from build123d import *

# Parameters (mm, degrees)
BOSS_EXTRUDE2_DEPTH = 8
SKETCH5_R           = 2.1
CUT_EXTRUDE1_DEPTH  = 130.846239099
FILLET1_R           = 8
SKETCH6_R           = 1
CUT_EXTRUDE2_DEPTH  = 7
BOSS_EXTRUDE3_DEPTH = 10
FILLET2_R           = 2
SKETCH9_W           = 4
SKETCH9_H           = 4
BOSS_EXTRUDE4_DEPTH = 21
SKETCH10_W          = 34
SKETCH10_H          = 4
BOSS_EXTRUDE5_DEPTH = 4
FILLET3_R           = 2
FILLET4_R           = 1
SKETCH11_R          = 1.95
CUT_EXTRUDE3_DEPTH  = 132.988809405


with BuildPart() as part:
    # Sketch3 → Boss-Extrude2 (new body)
    with BuildSketch(Plane(origin=(0, 0, 0), x_dir=(1, 0, 0), z_dir=(0, 1, 0))):
        Polygon((-66.423008775, -50), (-66.423008775, 50), (-15, 111.28355545), (15, 111.28355545), (66.423008775, 50), (66.423008775, -50), (15, -111.28355545), (-15, -111.28355545), align=None)
    extrude(amount=BOSS_EXTRUDE2_DEPTH)

    # Sketch5 → Cut-Extrude1 (cut, through all)
    with BuildSketch(Plane(origin=(0, 8, 0), x_dir=(1, 0, 0), z_dir=(0, 1, 0))):
        with Locations(Location((0, -106.28355545, 0), (0, 0, 270))):
            Circle(SKETCH5_R)
        with Locations(Location((-61.423008775, -48.180148829, 0), (0, 0, 270))):
            Circle(SKETCH5_R)
        with Locations(Location((0, 106.28355545, 0), (0, 0, 90))):
            Circle(SKETCH5_R)
        with Locations(Location((-61.423008775, 48.180148829, 0), (0, 0, 90))):
            Circle(SKETCH5_R)
        with Locations(Location((61.423008775, 48.180148829, 0), (0, 0, 270))):
            Circle(SKETCH5_R)
        with Locations(Location((61.423008775, -48.180148829, 0), (0, 0, 90))):
            Circle(SKETCH5_R)
    extrude(amount=-CUT_EXTRUDE1_DEPTH, mode=Mode.SUBTRACT)

    # Fillet1
    fillet1_edges = [part.edges().sort_by_distance(p)[0] for p in [
        (-66.423008775, 4, 50),
        (-66.423008775, 4, -50),
        (-15, 4, -111.28355545),
        (15, 4, -111.28355545),
        (66.423008775, 4, -50),
        (66.423008775, 4, 50),
        (15, 4, 111.28355545),
        (-15, 4, 111.28355545),
    ]]
    fillet(fillet1_edges, radius=FILLET1_R)

    # Sketch6 → Cut-Extrude2 (cut)
    with BuildSketch(Plane(origin=(0, 8, 0), x_dir=(1, 0, 0), z_dir=(0, 1, 0))):
        with Locations(Location((-44.948008775, -3.34355545, 0), (0, 0, 270))):
            Circle(SKETCH6_R)
        with Locations(Location((-44.948008775, -59.22355545, 0), (0, 0, 270))):
            Circle(SKETCH6_R)
        with Locations(Location((-25.898008775, -59.22355545, 0), (0, 0, 90))):
            Circle(SKETCH6_R)
        with Locations(Location((-25.898008775, -3.34355545, 0), (0, 0, 90))):
            Circle(SKETCH6_R)
        with Locations(Location((44.948008775, -59.22355545, 0), (0, 0, 90))):
            Circle(SKETCH6_R)
        with Locations(Location((25.898008775, -59.22355545, 0), (0, 0, 270))):
            Circle(SKETCH6_R)
        with Locations(Location((44.948008775, -3.34355545, 0), (0, 0, 90))):
            Circle(SKETCH6_R)
        with Locations(Location((25.898008775, -3.34355545, 0), (0, 0, 270))):
            Circle(SKETCH6_R)
    extrude(amount=-CUT_EXTRUDE2_DEPTH, mode=Mode.SUBTRACT)

    # Sketch8 → Boss-Extrude3 (add)
    with BuildSketch(Plane(origin=(0, 8, 0), x_dir=(1, 0, 0), z_dir=(0, 1, 0))):
        Polygon((8.295310149, 79.28355545), (11.295310149, 79.28355545), (11.295310149, 8.28355545), (29.895310149, 8.28355545), (29.895310149, 79.28355545), (32.895310149, 79.28355545), (32.895310149, 5.28355545), (8.295310149, 5.28355545), align=None)
    extrude(amount=BOSS_EXTRUDE3_DEPTH)

    # Fillet2
    fillet2_edges = [part.edges().sort_by_distance(p)[0] for p in [
        (8.295310149, 8, -42.28355545),
        (20.595310149, 8, -5.28355545),
        (32.895310149, 8, -42.28355545),
        (31.395310149, 8, -79.28355545),
        (9.795310149, 8, -79.28355545),
    ]]
    fillet(fillet2_edges, radius=FILLET2_R)

    # Sketch9 → Boss-Extrude4 (add)
    with BuildSketch(Plane(origin=(0, 8, 0), x_dir=(1, 0, 0), z_dir=(0, 1, 0))):
        with Locations((-44.423008775, 41.28355545)):
            Rectangle(SKETCH9_W, SKETCH9_H)
        with Locations((-14.423008775, 41.28355545)):
            Rectangle(SKETCH9_W, SKETCH9_H)
    extrude(amount=BOSS_EXTRUDE4_DEPTH)

    # Sketch10 → Boss-Extrude5 (add)
    with BuildSketch(Plane(origin=(0, 29, 0), x_dir=(1, 0, 0), z_dir=(0, 1, 0))):
        with Locations((-29.423008775, 41.28355545)):
            Rectangle(SKETCH10_W, SKETCH10_H)
    extrude(amount=BOSS_EXTRUDE5_DEPTH)

    # Fillet3
    fillet3_edges = [part.edges().sort_by_distance(p)[0] for p in [
        (-44.423008775, 8, -43.28355545),
        (-46.423008775, 8, -41.28355545),
        (-44.423008775, 8, -39.28355545),
        (-12.423008775, 8, -41.28355545),
        (-14.423008775, 8, -43.28355545),
        (-14.423008775, 8, -39.28355545),
        (-46.423008775, 33, -41.28355545),
        (-12.423008775, 33, -41.28355545),
    ]]
    fillet(fillet3_edges, radius=FILLET3_R)

    # Fillet4
    fillet4_edges = [part.edges().sort_by_distance(p)[0] for p in [
        (8.295310149, 18, -42.28355545),
        (20.595310149, 18, -5.28355545),
        (32.895310149, 18, -42.28355545),
    ]]
    fillet(fillet4_edges, radius=FILLET4_R)

    # Sketch11 → Cut-Extrude3 (cut, through all)
    with BuildSketch(Plane(origin=(0, 8, 0), x_dir=(1, 0, 0), z_dir=(0, 1, 0))):
        with Locations(Location((12.2, 0, 0), (0, 0, 270))):
            Circle(SKETCH11_R)
        with Locations(Location((-12.2, 0, 0), (0, 0, 270))):
            Circle(SKETCH11_R)
    extrude(amount=-CUT_EXTRUDE3_DEPTH, mode=Mode.SUBTRACT)


solid = part.part
Input: part model. Units: mm. Frame: model coordinates. A direction names the side the tool comes from. Coordinates: 2 decimals unless noted, no trailing zeros. Order: outer loops, then holes, each group sorted by start corner. A loop starts at its lowest first (then second) coordinate and runs counter-clockwise, first axis right, second up. Notation, with made-up numbers: M -11,80.25 L -4,80.25 A6 ccw -4,90.25 Z; hole C 17,-30.5 d2. An arc over 180 degrees is marked long. One line per question, with ' | ' between items.
Item 1: Section B-B (y = 13). Output: boundary loops of the cut face in (x, z), then the cut area to 3 significant figures.
Geometry results:
outline: M -46.42,-43.28 L -42.42,-43.28 L -42.42,-39.28 L -46.42,-39.28 Z; M -16.42,-43.28 L -12.42,-43.28 L -12.42,-39.28 L -16.42,-39.28 Z; M 8.3,-79.28 L 11.3,-79.28 L 11.3,-8.28 L 29.9,-8.28 L 29.9,-79.28 L 32.9,-79.28 L 32.9,-5.28 L 8.3,-5.28 Z | area: 532 mm^2
Item 2: Reachability of faces 1 (the flat face through (-42.423, 18, -41)), 2 (the cylindrical face through (-65.954, 4.056, -49.788)), 3 (the flat face through (-46.423, 20, -41)), 4 (the flat face through (20, 13, -8.284)), 5 (the flat face through (-30, 32, -39.284)) from +Z, -Z, +X, -X, +Y, -Y: full face, straight path, thin tool, end or side. Return the list, or none.
Geometry results:
face 1: +Z, -Z | face 2: -Z, -X, +Y, -Y | face 3: +Z, -Z, -X, +Y | face 4: -Z, +Y | face 5: +Z, -X, +Y
Item 3: Pin query (flat end, axial travel): pin 1 (10 mm diameter, centred on x = 2.5, y = 11, fed in from +Z); pin 2 (2.5 mm diameter, centred on y = 15, z = -40.5, fed in from -X); pin 3 (10 mm diameter, centred on x = 35.5, y = 20.5, fed in from +Z); pin 4 (6.5 mm diameter, centred on x = -61.42, z = -48.18, fed in from +Y). Return the tip coordinate at first contact, or that it passes through.
Geometry results:
pin 1: stops at z = 111.28 | pin 2: stops at x = -46.42 | pin 3: stops at z = -5.28 | pin 4: stops at y = 8
Item 4: Section D-D (z = -67). Output: boundary loops of the cut face in (x, y), then the cut area to 3 significant figures.
Geometry results:
outline: M -52.16,0 L 52.16,0 L 52.16,8 L 34.9,8 A2 cw 32.9,10 L 32.9,17 A1 ccw 31.9,18 L 29.9,18 L 29.9,8 L 11.3,8 L 11.3,18 L 9.3,18 A1 ccw 8.3,17 L 8.3,10 A2 cw 6.3,8 L -52.16,8 Z | area: 896 mm^2
Item 5: Draft query along Z for faces 6 (the flat face through (1, 0, -2)), 7 (the flat face through (21, 13, -5.284)), 8 (the cylindrical face through (63.47, 4.06, 48.64)), 9 (the cylindrical face through (-63.505, 4.056, -47.907)). Return one class per face: released by +Z, released by -Z, zero draft, split by the parting line, or undercut.
Geometry results:
face 6: zero draft | face 7: released by +Z | face 8: undercut | face 9: undercut
Item 6: Section C-C (y = 26.5). Output: boundary loops of the cut face in (x, z).
Geometry results:
outline: M -46.42,-43.28 L -42.42,-43.28 L -42.42,-39.28 L -46.42,-39.28 Z; M -16.42,-43.28 L -12.42,-43.28 L -12.42,-39.28 L -16.42,-39.28 Z
Item 7: Ray query, line 1 along X through (y, z) = (5, 4); line 2 along Y through (x, z) = (-60.5, 11.5); line 3 along Z through (x, y) = (19, 14.5). Return the intervals inside material, ascending.
Geometry results:
line 1: x = -66.42 to -45.7, -44.19 to -26.65, -25.14 to 25.14, 26.65 to 44.19, 45.7 to 66.42 | line 2: y = 0 to 8 | line 3: z = -8.28 to -5.28
Item 8: Section A-A (x = 0). Output: boundary loops of the cut face in (y, z).
Geometry results:
outline: M 0,-111.28 L 8,-111.28 L 8,-108.38 L 0,-108.38 Z; M 0,-104.18 L 8,-104.18 L 8,104.18 L 0,104.18 Z; M 0,108.38 L 8,108.38 L 8,111.28 L 0,111.28 Z
